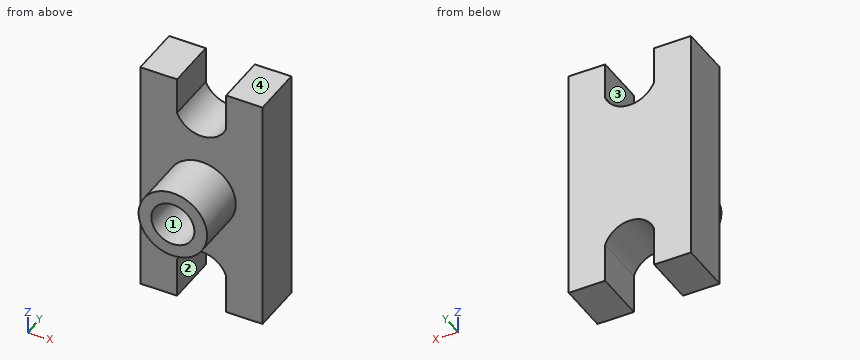
from build123d import *

# Parameters (mm, degrees)
F1_DEPTH = 25.4
F2_R     = 16.682026
F2_R_2   = 10.500829
F3_DEPTH = 25.4


with BuildPart() as f1:
    # F0 (on Front) → F1 (new body)
    with BuildSketch(Plane.XZ):
        with BuildLine():
            Line((-23.929596, 61.36547), (-41.840091, 61.36547))
            Line((-41.840091, 61.36547), (-41.840091, -54.025102))
            Line((-41.840091, -54.025102), (-23.929596, -54.025102))
            Line((-23.929596, -54.025102), (-23.929596, -34.940146))
            ThreePointArc((-23.929596, -34.940146), (-11.964798, -26.243898), (0, -34.940146))
            Line((0, -34.940146), (0, -54.025102))
            Line((0, -54.025102), (17.763687, -54.025102))
            Line((17.763687, -54.025102), (17.763687, 61.36547))
            Line((17.763687, 61.36547), (0, 61.36547))
            Line((0, 61.36547), (0, 43.454971))
            ThreePointArc((0, 43.454971), (-11.964798, 35.3963), (-23.929596, 43.454971))
            Line((-23.929596, 43.454971), (-23.929596, 61.36547))
        make_face()
    extrude(amount=F1_DEPTH)

    # F2 (on face) → F3 (join)
    with BuildSketch(Plane.XZ.offset(25.4)):
        with Locations((-11.964798, 4.991449)):
            Circle(F2_R)
        with Locations((-11.964798, 4.991449)):
            Circle(F2_R_2, mode=Mode.SUBTRACT)
    extrude(amount=F3_DEPTH)


solid = f1.part
Source: CAD feature listing. Evaluate the final solid. Frame: model axes, mm. Face numbers are marked on the shaded views. A direction names the side the tool comes from. Give positions to 0.01 mm unless a question says otherwise; leave off trailing zeros. Write each loop counter-clockwise with the first axis right and the second up, starting at its lowest first coordinate (ties: lowest second). Pieces come first, ordered by that corner, then holes. Notation, with made-up numbers: M -16.75,66 L -4.75,66 A38 cw -4.75,104 Z; hole C 12,-6.5 d7. An arc over 180 degrees is marked long. Return JSON: item names as keys, results as strings. Group by question number.
1) Pin query (flat end, axial travel): P1, Ø1.5, axis at x = -8.5, y = -12.5, coming from the +Z side; P2, Ø3, axis at x = -16.5, y = -37.5, coming from the +Z side; P3, Ø10.5, axis at x = -12, z = 6, coming from the -Y side. Return the tip coordinate at first contact, or that it passes through.
2) Cut plane D-D, the plane z = 29. Output: boundary loops of the cut face in (x, y).
3) Cut plane A-A, the plane z = -45. Output: boundary loops of the cut face in (x, y), plus the area to 3 significant figures.
4) Cut plane C-C, the plane x = -6.5. Output: boundary loops of the cut face in (y, z), plus the area to 3 significant figures.
5) Set-up query: the marked faces 1, 2, 3 and 4. Return all of +Z, -Z, +X, -X, +Y, -Y with unobstructed straight access to the full face (end or side cutting, diameter ignored); none if empty.
6) Material intervals for line 1 along X through (y, z) = (-21.5, -47); line 2 along Y through (x, z) = (-32.5, -20.5); line 3 along X through (y, z) = (-7.5, 43), sorted ascending. Write a range as [from, to].
7) Cut plane B-B, the plane y = -16. Output: boundary loops of the cut face in (x, z), plus the area to 3 significant figures.
Recorded:
{
 "1": {"P1": "stops at z = 36.1", "P2": "stops at z = 21.4", "P3": "stops at y = -25.4"},
 "2": {"outline": "M -41.84,-25.4 L 17.76,-25.4 L 17.76,0 L -41.84,0 Z"},
 "3": {"outline": "M -41.84,-25.4 L -23.93,-25.4 L -23.93,0 L -41.84,0 Z; M 0,-25.4 L 17.76,-25.4 L 17.76,0 L 0,0 Z", "area": "906 mm²"},
 "4": {"outline": "M -50.8,-10.77 L -25.4,-10.77 L -25.4,-27.49 L 0,-27.49 L 0,36.61 L -25.4,36.61 L -25.4,20.75 L -50.8,20.75 L -50.8,13.96 L -25.4,13.96 L -25.4,-3.98 L -50.8,-3.98 Z", "area": "1,970 mm²"},
 "5": {"face 1": "-Y", "face 2": "-Z, +Y, -Y", "face 3": "+Z, +Y, -Y", "face 4": "+Z, +X, -X, +Y, -Y"},
 "6": {"line 1": "x = [-41.84, -23.93], [0, 17.76]", "line 2": "y = [-25.4, 0]", "line 3": "x = [-41.84, -23.73], [-0.19, 17.76]"},
 "7": {"outline": "M -41.84,-54.03 L -23.93,-54.03 L -23.93,-34.94 A12.58 cw 0,-34.94 L 0,-54.03 L 17.76,-54.03 L 17.76,61.37 L 0,61.37 L 0,43.45 A12.91 cw -23.93,43.45 L -23.93,61.37 L -41.84,61.37 Z", "area": "5,700 mm²"}
}
